For this review, take the finished solid that the model builds, in its own axes (mm). Face numbers are marked on the shaded views. A direction names the side the tool comes from. Give positions to 0.01 mm unless a question says otherwise; leave off trailing zeros.
Item 1: Machinability: for the marked faces 1 and 2, which of the approach directions +Z, -Z, +X, -X, +Y, -Y give a long, thin tool a straight path to every point of the face, cutting with its end or side? Answer none if there is none.
Item 2: For probe 1 along Y at (x, z) = (22.5, 0.25); probe 2 along X at (y, z) = (8.7, -9); probe 3 along Z at (x, y) = (24.5, 8.75), list the stretches that pass through material, from the lowest coordinate up.
Item 3: For P1, Ø8, axis at x = 39.5, z = -9.5, coming from the +Y side; P2, Ø1.5, axis at x = 40.5, z = -10.5, coming from the -Y side; P3, Ø2, axis at x = 30.5, y = 7.5, coming from the -Z side; P4, Ø3, axis at x = 31, z = 11.5, coming from the -Y side, all flat-tipped, find the tip position at first contact; note any pin that passes through.
```python
from build123d import *

# Parameters (mm, degrees)
SCALE1_SCALE = 0.5
SCALE2_SCALE = 0.3
SCALE3_SCALE = 0.5
SCALE5_SCALE = 5


with BuildPart() as part:
    # Sketch1 → Revolve1 (revolve)
    with BuildSketch(Plane.XY, mode=Mode.PRIVATE) as revolve1_sk:
        with BuildLine():
            Line((-2.258036414, 14.369211187), (30.108325784, 14.369211187))
            Line((30.108325784, 14.369211187), (30.108325784, 2.156708547))
            Line((30.108325784, 2.156708547), (-2.258036414, 2.156708547))
            ThreePointArc((-2.258036414, 2.156708547), (-8.364287734, 8.262959867), (-2.258036414, 14.369211187))
        make_face()
    revolve(revolve1_sk.sketch.rotate(Axis((30.290952568, 14.369211187, 0), (-0.004261675171453159, -0.9999909190211345, 0)), 180), axis=Axis((30.290952568, 14.369211187, 0), (-0.004261675171453159, -0.9999909190211345, 0)))


with BuildPart() as part_1:
    # Scale1: scaled about (30.264488075, 8.159387293, 0)
    add(part.part.scale(SCALE1_SCALE).moved(Location((15.132244037, 4.079693646, 0))))


with BuildPart() as part_2:
    # Scale2: scaled about (30.264488075, 8.159387293, 0)
    add(part_1.part.scale(SCALE2_SCALE).moved(Location((21.185141652, 5.711571105, 0))))


with BuildPart() as part_3:
    # Scale3: scaled about (30.264488075, 8.159387293, 0)
    add(part_2.part.scale(SCALE3_SCALE).moved(Location((15.132244037, 4.079693646, 0))))


with BuildPart() as part_4:
    # Scale5: scaled about (30.264488075, 8.159387293, 0)
    add(part_3.part.scale(SCALE5_SCALE).moved(Location((-121.0579523, -32.637549172, 0))))


solid = part_4.part
```
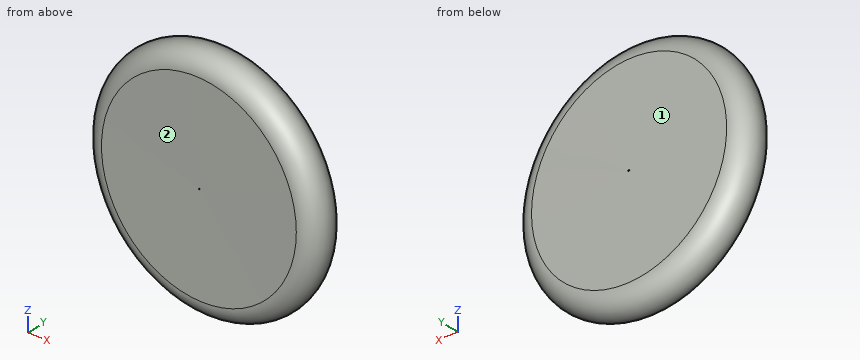
Resolved:
1. face 1: +X, +Y
1. face 2: -X, -Y
2. probe 1: y = 5.91 to 10.49
2. probe 2: x = 18.99 to 41.51
2. probe 3: z = -13.21 to 13.21
3. P1: stops at y = 10.42
3. P2: stops at y = 6.6
3. P3: stops at z = -14.49
3. P4: stops at y = 5.85
